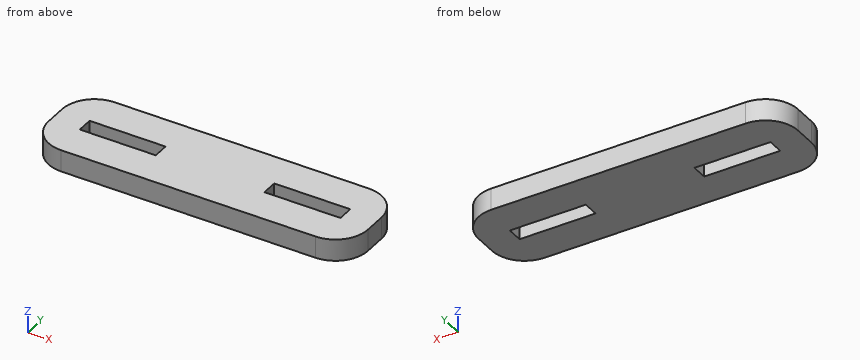
```python
from build123d import *

# Parameters (mm, degrees)
SKETCH1_W           = 7
SKETCH1_H           = 1.46
BOSS_EXTRUDE1_DEPTH = 2


with BuildPart() as part:
    # Sketch1 → Boss-Extrude1 (new body)
    with BuildSketch(Plane.XY):
        with BuildLine():
            Line((-31.064544979, 27.784009845), (-7.664544979, 27.784009845))
            ThreePointArc((-7.664544979, 27.784009845), (-5.543224635, 26.905330188), (-4.664544979, 24.784009845))
            Line((-4.664544979, 24.784009845), (-4.664544979, 22.784009845))
            ThreePointArc((-4.664544979, 22.784009845), (-5.543224635, 20.662689501), (-7.664544979, 19.784009845))
            Line((-7.664544979, 19.784009845), (-31.064544979, 19.784009845))
            ThreePointArc((-31.064544979, 19.784009845), (-33.185865322, 20.662689501), (-34.064544979, 22.784009845))
            Line((-34.064544979, 22.784009845), (-34.064544979, 24.784009845))
            ThreePointArc((-34.064544979, 24.784009845), (-33.185865322, 26.905330188), (-31.064544979, 27.784009845))
        make_face()
        with Locations((-27.864544979, 23.784009845)):
            Rectangle(SKETCH1_W, SKETCH1_H, mode=Mode.SUBTRACT)
        with Locations((-10.864544979, 23.784009845)):
            Rectangle(SKETCH1_W, SKETCH1_H, mode=Mode.SUBTRACT)
    extrude(amount=BOSS_EXTRUDE1_DEPTH)


solid = part.part
```
Here's how the part is built. I have some questions about the finished solid (model axes, mm). Give positions to 0.01 mm unless a question says otherwise; leave off trailing zeros. Loops run counter-clockwise (first coordinate to the right, second up) from the corner with the lowest first, then second, coordinate; pieces in that order, holes last. Notation, with made-up numbers: M -16,-4.75 L 14,-4.75 A21 ccw 14,1.25 Z; hole C -20.5,-21.75 d3. An arc over 180 degrees is marked long. Return JSON: item names as keys, results as strings.
Item 1: Imagine slicing it at B-B on z = 0.7. List the corners of the cut face in (x, y) for me, then the cut area to 3 significant figures.
A:
{"outline": "M -34.06,22.78 A3 ccw -31.06,19.78 L -7.66,19.78 A3 ccw -4.66,22.78 L -4.66,24.78 A3 ccw -7.66,27.78 L -31.06,27.78 A3 ccw -34.06,24.78 Z; hole M -31.36,23.05 L -24.36,23.05 L -24.36,24.51 L -31.36,24.51 Z; hole M -14.36,23.05 L -7.36,23.05 L -7.36,24.51 L -14.36,24.51 Z", "area": "207 mm^2"}
Item 2: Imagine slicing it at A-A on x = -13. List the corners of the cut face in (y, z) for me, then the cut area to 3 significant figures.
A:
{"outline": "M 19.78,0 L 23.05,0 L 23.05,2 L 19.78,2 Z; M 24.51,0 L 27.78,0 L 27.78,2 L 24.51,2 Z", "area": "13.1 mm^2"}
Item 3: Imagine slicing it at C-C on y = 26.5. List the corners of the cut face in (x, z) for me, then the cut area to 3 significant figures.
A:
{"outline": "M -33.53,0 L -5.2,0 L -5.2,2 L -33.53,2 Z", "area": "56.6 mm^2"}
Item 4: Imagine slicing it at D-D on x = -6.5. List the corners of the cut face in (y, z) for me, then the cut area to 3 significant figures.
A:
{"outline": "M 20.02,0 L 27.55,0 L 27.55,2 L 20.02,2 Z", "area": "15.1 mm^2"}
Item 5: Please list where these lines run through material, in increasing order: line 1 (X direction, y = 23.5, z = 0.8); line 2 (Y direction, x = -11.75, z = 0.95); line 3 (X direction, y = 26.75, z = 1.65).
A:
{"line 1": "x = -34.06 to -31.36, -24.36 to -14.36, -7.36 to -4.66", "line 2": "y = 19.78 to 23.05, 24.51 to 27.78", "line 3": "x = -33.33 to -5.4"}
